from build123d import *

# Parameters (mm, degrees)
EXTRUDE_THIN1_DEPTH = 25.4
BOSS_EXTRUDE1_REACH = 633.439
SKETCH3_W           = 25.4
SKETCH3_H           = 3.175
BOSS_EXTRUDE2_REACH = 587.221
SKETCH4_W           = 25.4
SKETCH4_H           = 3.175


with BuildPart() as part:
    # Sketch2 → Extrude-Thin1 (new body)
    with BuildSketch(Plane.XY):
        with BuildLine():
            ThreePointArc((-128.959094117, -567.323540773), (-123.788950473, -572.673268248), (-130.145681643, -576.538748578))
            Line((-130.145681643, -576.538748578), (-302.042094367, -513.783924281))
            ThreePointArc((-302.042094367, -513.783924281), (-325.948053636, -436.522751042), (-245.108142892, -434.136832006))
            Line((-245.108142892, -434.136832006), (-198.273248153, -492.098506685))
            ThreePointArc((-198.273248153, -492.098506685), (-185.155706812, -490.955524281), (-191.14596289, -479.229777749))
            Line((-191.14596289, -479.229777749), (-191.527323999, -482.381791186))
            ThreePointArc((-191.527323999, -482.381791186), (-187.933170352, -489.417239105), (-195.803695157, -490.103028547))
            Line((-195.803695157, -490.103028547), (-242.638589895, -432.141353869))
            ThreePointArc((-242.638589895, -432.141353869), (-328.530995061, -434.676392845), (-303.130913338, -516.76638941))
            Line((-303.130913338, -516.76638941), (-131.234500614, -579.521213708))
            ThreePointArc((-131.234500614, -579.521213708), (-120.639948663, -573.078746491), (-129.256854737, -564.162534033))
            Line((-129.256854737, -564.162534033), (-128.959094117, -567.323540773))
        make_face()
    extrude(amount=EXTRUDE_THIN1_DEPTH)

    # Boss-Extrude1: up to this plane
    boss_extrude1_end = Plane(origin=(-242.638589895, -432.141353869, 25.4), z_dir=(-0.7778119673882409, -0.6284970512163396, 0))
    # Sketch3 → Boss-Extrude1 (add, up to the surface)
    with BuildSketch(Plane(origin=(-131.24290391, 15.879037441, 0), x_dir=(0, 0, 1), z_dir=(-0.9927601375164752, 0.12011373509415744, 0)), mode=Mode.PRIVATE) as boss_extrude1_sk1:
        with Locations((12.7, -500.306975611)):
            Rectangle(SKETCH3_W, SKETCH3_H)
    boss_extrude1_tool1 = split(extrude(boss_extrude1_sk1.sketch, amount=BOSS_EXTRUDE1_REACH, mode=Mode.PRIVATE), bisect_by=boss_extrude1_end, keep=Keep.BOTH, mode=Mode.PRIVATE)
    add(boss_extrude1_tool1.solids().sort_by_distance((-191.336643, -480.805784, 12.7))[0])

    # Boss-Extrude2: up to this plane
    boss_extrude2_end = Plane(origin=(-302.042094367, -513.783924281, 25.4), z_dir=(0.3429351088975487, 0.9393590959188219, 0))
    # Sketch4 → Boss-Extrude2 (add, up to the surface)
    with BuildSketch(Plane(origin=(-180.795608077, -17.030590821, 0), x_dir=(0, 0, 1), z_dir=(-0.9955926741540518, -0.09378287248098222, 0)), mode=Mode.PRIVATE) as boss_extrude2_sk1:
        with Locations((12.7, -551.14150679)):
            Rectangle(SKETCH4_W, SKETCH4_H)
    boss_extrude2_tool1 = split(extrude(boss_extrude2_sk1.sketch, amount=BOSS_EXTRUDE2_REACH, mode=Mode.PRIVATE), bisect_by=boss_extrude2_end, keep=Keep.BOTH, mode=Mode.PRIVATE)
    add(boss_extrude2_tool1.solids().sort_by_distance((-129.107974, -565.743037, 12.7))[0])


solid = part.part
Work out the finished part from the listing and answer in its coordinate system (mm). A direction names the side the tool comes from. Round coordinates to 2 decimals unless told otherwise and drop trailing zeros. Loops run counter-clockwise (first coordinate to the right, second up) from the corner with the lowest first, then second, coordinate; pieces in that order, holes last. Notation, with made-up numbers: (-30, 71.5) - (11, 71.5) arc R18 cw to (11, 100.5) - close; hole circle Ø4 at (1, 43). An arc over 180 degrees is marked (long way). Use one line per item in the form item = value. Start each with the question number.
(1) Find section C-C on x = -254. Determine the outline of the cut face in (y, z), and give its area (3 significant figures).
(2) Which of the six approach directions +Z, -Z, +X, -X, +Y, -Y give full straight-line access (tool end or side, diameter ignored) to faces 4 (the face through (-142.89, -565.447, 12.522)), 5 (the face through (-210, -476, 25.4)), 6 (the face through (-222.02, -462.71, 12.52))?
(3) Find section B-B on x = -307. Determine the outline of the cut face in (y, z), and give its area (3 significant figures).
(4) Find section A-A on z = 5.75. Give the number of separate pieces and of enclosed holes in the cut face, and give its area (3 significant figures).
(5) Determine the mould class of faces 1 (the face through (-120.67, -573.28, 12.52)), 2 (the face through (-187.87, -489.3, 12.52)), 3 (the face through (-218.4, -547.7, 12.5)) for opening direction Y: +Y half, -Y half, draft (parallel to the pull), parting line (faces both ways), or undercut.
(6) Consider line 1 (Y direction, x = -282, z = 9.25); line 2 (Y direction, x = -327, z = 4.75); line 3 (X direction, y = -493, z = 11.5). Determine where each line is inside the solid, lowest interval first.
(7) Flat-ended cylindrical pins translate along their axes: P1, Ø8.5, axis at x = -128.51, y = -572.07, coming from the -Z side; P2, Ø8, axis at x = -275, z = 19, coming from the -Y side; P3, Ø15, axis at x = -192.1, y = -487.11, coming from the -Z side; P4, Ø3, axis at y = -443.5, z = 14.5, coming from the +X side. Find the tip coordinate at first contact, or state that the pin passes through.
(8) Find section D-D on y = -534.5. Determine the outline of the cut face in (x, z).
Answer list:
q1.outline = (-534.7, 0) - (-531.32, 0) - (-531.32, 25.4) - (-534.7, 25.4) - close; (-425.53, 0) - (-421.62, 0) - (-421.62, 25.4) - (-425.53, 25.4) - close
q1.area = 185 mm^2
q2.face_4 = +Z, -Z, +Y
q2.face_5 = +Z, +X, -X, +Y, -Y
q2.face_6 = +Z, -Z
q3.outline = (-515.18, 0) - (-511.67, 0) - (-511.67, 25.4) - (-515.18, 25.4) - close; (-420.46, 0) - (-416.95, 0) - (-416.95, 25.4) - (-420.46, 25.4) - close
q3.area = 178 mm^2
q4.separate_pieces = 1
q4.enclosed_holes = 2
q4.area = 1,700 mm^2
q5.face_1 = parting line
q5.face_2 = undercut
q5.face_3 = -Y half
q6.line_1 = -524.48 to -521.1, -415.33 to -412.15
q6.line_2 = -499.49 to -494.08, -438.05 to -432.64
q6.line_3 = -331.39 to -327.69, -197.42 to -186.78
q7.P1 = through
q7.P2 = -528.5
q7.P3 = 0
q7.P4 = -232.25
q8.outline = (-254.56, 0) - (-245.3, 0) - (-245.3, 25.4) - (-254.56, 25.4) - close
